Design review of the part built by this model. Coordinates are the model's own, in mm. A direction names the side the tool comes from. Coordinates: 2 decimals unless noted, no trailing zeros. Order: outer loops, then holes, each group sorted by start corner. A loop starts at its lowest first (then second) coordinate and runs counter-clockwise, first axis right, second up. Notation, with made-up numbers: (-17, 72.25) - (22, 72.25) arc R30 cw to (22, 105.25) - close; hole circle Ø11 at (-19.75, 11.25). An arc over 180 degrees is marked (long way). Write item = value, one per line. Start each with the question number.
```python
from build123d import *

# Parameters (mm, degrees)
F1_DEPTH = 30
F2_R     = 29.99999
F3_R     = 15
F4_DEPTH = 15
F6_R     = 5
F7_DEPTH = 20


# Not quite as in the source:
# - a fillet or chamfer is up to 0.001 mm smaller than in the source, because OpenCascade refuses the exact size


with BuildPart() as f1:
    # F0 (on Front) → F1 (new body, symmetric)
    with BuildSketch(Plane.XZ):
        Polygon((-100, 0), (0, 0), (0, 35), (-20, 35), (-20, 15), (-100, 15), align=None)
    extrude(amount=F1_DEPTH, both=True)

    # F2 (radius 30 in the source; OpenCascade refuses exactly that, so slightly less here)
    f2_edges = [f1.edges().sort_by_distance(p)[0] for p in [
        (-100, -30, 7.5),
        (-100, 30, 7.5),
    ]]
    fillet(f2_edges, radius=F2_R)

    # F3 (on face) → F4 (cut, through all)
    with BuildSketch(Plane.XY.offset(15)):
        with Locations((-70, 0)):
            Circle(F3_R)
    extrude(amount=-F4_DEPTH, mode=Mode.SUBTRACT)

    # F5: F1 across plane


with BuildPart() as f1_1:
    add(f1.part)
    add(f1.part.mirror(Plane.XY))

    # F6 (on face) → F7 (cut, through all)
    with BuildSketch(Plane.YZ):
        with BuildLine():
            ThreePointArc((-20, -30), (-16.4644660941, -28.5355339059), (-15, -25))
            ThreePointArc((-15, -25), (-23.5355339059, -21.4644660941), (-20, -30))
        make_face()
        with Locations((-20, 25)):
            Circle(F6_R)
        with Locations((20, -25)):
            Circle(F6_R)
        with Locations((20, 25)):
            Circle(F6_R)
    extrude(amount=-F7_DEPTH, mode=Mode.SUBTRACT)


solid = f1_1.part
```
Item 1: For line 1 (Z direction, x = -15.5, y = -20); line 2 (Y direction, x = -70, z = 0.25); line 3 (Z direction, x = -78, y = -25), list the stretches that pass through material, from the lowest coordinate up.
Item 2: For faces 1 (the flat face through (-51, 0, -15)), 2 (the flat face through (-20, 0, 25)), 3 (the flat face through (0, 0, 0)), list the 3-axis set-ups (+Z, -Z, +X, -X, +Y, -Y) from which the entire face can be reached by the end or side of a thin tool; tool diameter is ignored.
Item 3: Add section D-D on y = 22.5. Give the boundary of the cut face in (x, z).
Item 4: Add section B-B on z = 25. Give the boundary of the cut face in (x, y), plus the area to 3 significant figures.
Item 5: Add section C-C on y = -10.5. Give the boundary of the cut face in (x, z), plus the area to 3 significant figures.
Item 6: Mouldability with a two-part tool opening along Y and no side actions: class faces 4 (the flat face through (-28, -30, 0)), 5 (the flat face through (-10, 0, 35)), 6 (the cylindrical face through (-91.445, 20.979, 0.21)), 7 (the cylindrical face through (-9.86, -21.08, 20.12)) as +Y half, -Y half, draft (parallel to the pull), parting line (faces both ways), or undercut.
Item 7: Add section A-A on x = -8. Give the boundary of the cut face in (y, z).
Item 8: For P1, Ø2, axis at x = -77.5, y = -12, coming from the -Z side; P2, Ø10, axis at x = -40, y = -13.5, coming from the +Z side; P3, Ø16, axis at y = -11, z = -21, coming from the -X side, all flat-tipped, find the tip position at first contact; note any pin that passes through.
Worked out:
q1.line_1 = -35 to -30, -20 to 20, 30 to 35
q1.line_2 = -30 to -15, 15 to 30
q1.line_3 = -15 to 15
q2.face_1 = -Z, -X, +Y, -Y
q2.face_2 = +Z, -X, +Y, -Y
q2.face_3 = +Z, -Z, +X, +Y, -Y
q3.outline = (-89.84, -15) - (-20, -15) - (-20, -20.67) - (0, -20.67) - (0, 20.67) - (-20, 20.67) - (-20, 15) - (-89.84, 15) - close; (-20, -35) - (0, -35) - (0, -29.33) - (-20, -29.33) - close; (-20, 29.33) - (0, 29.33) - (0, 35) - (-20, 35) - close
q4.outline = (-20, -30) - (0, -30) - (0, -25) - (-20, -25) - close; (-20, -15) - (0, -15) - (0, 15) - (-20, 15) - close; (-20, 25) - (0, 25) - (0, 30) - (-20, 30) - close
q4.area = 800 mm2
q5.outline = (-98.1, -15) - (-80.71, -15) - (-80.71, 15) - (-98.1, 15) - close; (-59.29, -15) - (-20, -15) - (-20, -35) - (0, -35) - (0, 35) - (-20, 35) - (-20, 15) - (-59.29, 15) - close
q5.area = 3,100 mm2
q6.face_4 = -Y half
q6.face_5 = draft
q6.face_6 = +Y half
q6.face_7 = undercut
q7.outline = (-30, -35) - (30, -35) - (30, 35) - (-30, 35) - close; hole circle Ø10 at (-20, -25); hole circle Ø10 at (-20, 25); hole circle Ø10 at (20, -25); hole circle Ø10 at (20, 25)
q8.P1 = -15
q8.P2 = 15
q8.P3 = -99.45
